Model file for the job. Use its own axes, mm. Face numbers are marked on the shaded views. A direction names the side the tool comes from. Round coordinates to 2 decimals unless told otherwise and drop trailing zeros. Write each loop counter-clockwise with the first axis right and the second up, starting at its lowest first coordinate (ties: lowest second). Pieces come first, ordered by that corner, then holes.
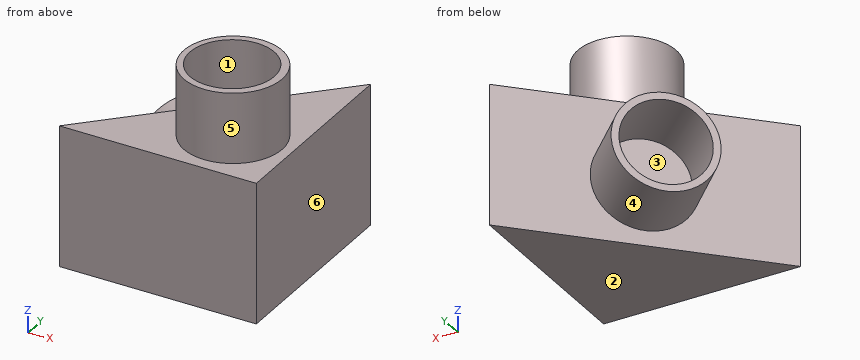
```python
from build123d import *

# Parameters (mm, degrees)
F1_DEPTH = 25.4
F3_R     = 8.89
F4_DEPTH = 12.7
F2_R     = 7.62
F5_DEPTH = 39.116
F6_R     = 8.89
F6_R_2   = 7.62
F7_DEPTH = 12.7


with BuildPart() as f1:
    # F0 (on Top) → F1 (new body)
    with BuildSketch(Plane.XY):
        Polygon((-24.6135034411, 35.56), (-60.1735034411, 0), (-24.6135034411, 0), align=None)
    extrude(amount=F1_DEPTH)

    # F3 (on face) → F4 (join)
    with BuildSketch(Plane.XY.offset(25.4)):
        with Locations((-35.3040769696, 11.1599909142)):
            Circle(F3_R)
    extrude(amount=F4_DEPTH)

    # F2 (on face) → F5 (cut)
    with BuildSketch(Plane.XY.offset(25.4)):
        with Locations((-35.4857780039, 11.2061388791)):
            Circle(F2_R)
    extrude(amount=F5_DEPTH, mode=Mode.SUBTRACT)

    # F6 (on face) → F7 (join)
    with BuildSketch(Plane(origin=(-30.0867517206, 30.0867517206, 0), x_dir=(-0.7071067812, -0.7071067812, 0), z_dir=(-0.7071067812, 0.7071067812, 0))):
        with Locations((17.4403432757, 11.6122188047)):
            Circle(F6_R)
        with Locations((17.4403432757, 11.6122188047)):
            Circle(F6_R_2, mode=Mode.SUBTRACT)
    extrude(amount=F7_DEPTH)


solid = f1.part
```
1) Wall check: probe 1 along Z at (x, y) = (-29.5, 8); probe 2 along X at (y, z) = (22, 7); probe 3 along X at (y, z) = (21, 14). Give the ranges that are in metal, low to high.
2) Which spindle directions (+Z, -Z, +X, -X, +Y, -Y) get a long thin tool onto all of the face, cutting with end or side? Do the marked faces 1, 2 and 3. Say none if no direction does.
3) Pull direction X, two halves, no side cores. Call the marked faces 4, 5 and 6: released by +X, released by -X, zero draft, split by the parting line, or undercut.
4) Flat gauge pins, fed straight in: pin 1 Ø1.5 at (x, y) = (-52.5, 24) entering from +Z; pin 2 Ø2 at (x, y) = (-32.5, 15) entering from -Z; pin 3 Ø4 at (x, z) = (-49, 16.5) entering from +Y; pin 4 Ø12 at (x, z) = (-48, 32) entering from +Y. Where does each tip first touch, or does it go through?
5) Cut at C-C on y = 10. List the corners of the cut face in (x, z).
6) Cut at B-B on x = -35.5. List the corners of the cut face in (y, z), and give its area (3 significant figures).
7) Cut at D-D on z = 32.5. List the corners of the cut face in (x, y), and give its area (3 significant figures).
8) Cut at A-A on z = 7. List the corners of the cut face in (x, y), and give its area (3 significant figures).
Result sheet:
1. probe 1: z = 0 to 25.4
1. probe 2: x = -56.13 to -55.24, -38.17 to -24.61
1. probe 3: x = -57.13 to -55.9, -39.17 to -24.61
2. face 1: +Z
2. face 2: -Z, +X, -X, +Y, -Y
2. face 3: none
3. face 4: undercut
3. face 5: split by the parting line
3. face 6: released by +X
4. pin 1: stops at z = 20.28
4. pin 2: stops at z = 0
4. pin 3: stops at y = 31.13
4. pin 4: stops at y = 17.01
5. outline: (-50.17, 0) - (-24.61, 0) - (-24.61, 25.4) - (-26.49, 25.4) - (-26.49, 38.1) - (-27.96, 38.1) - (-27.96, 25.4) - (-43.01, 25.4) - (-43.01, 38.1) - (-44.12, 38.1) - (-44.12, 25.4) - (-50.17, 25.4) - close
6. outline: (0, 0) - (24.67, 0) - (24.67, 25.4) - (20.05, 25.4) - (20.05, 38.1) - (18.83, 38.1) - (18.83, 25.4) - (3.59, 25.4) - (3.59, 38.1) - (2.27, 38.1) - (2.27, 25.4) - (0, 25.4) - close
6. area: 659 mm2
7. outline: circle Ø17.78 at (-35.3, 11.16); hole circle Ø15.24 at (-35.49, 11.21)
7. area: 65.9 mm2
8. outline: (-60.17, 0) - (-24.61, 0) - (-24.61, 35.56) - (-37.04, 23.13) - (-46.03, 32.11) - (-47.11, 31.02) - (-38.13, 22.04) - (-46.71, 13.47) - (-55.69, 22.45) - (-56.77, 21.36) - (-47.79, 12.38) - close
8. area: 671 mm2
